Read the model definition and answer for the solid it produces. Units are mm, in the model's axes. A direction names the side the tool comes from. Round coordinates to 2 decimals unless told otherwise and drop trailing zeros. Order: outer loops, then holes, each group sorted by start corner. A loop starts at its lowest first (then second) coordinate and runs counter-clockwise, first axis right, second up. Notation, with made-up numbers: M 66.5,-13 L 86.5,-13 A9 ccw 86.5,0 Z; hole C 23,24.5 d7. An arc over 180 degrees is marked long. Use one line per item in the form item = value. Start each with the question number.
from build123d import *

# Parameters (mm, degrees)
CHANFRO1_SIZE = 0.5
FILETE1_R     = 3


with BuildPart() as part:
    # Esboço1 → Revolução1 (revolve)
    with BuildSketch(Plane(origin=(0, 0, 0), x_dir=(0, 0, -1), z_dir=(1, 0, 0))):
        Polygon((23.5, 20), (20, 20), (9.495318128, -6), (14.495318128, -6), (25, 20), (29.5, 20), (29.5, 35), (21.5, 35), (21.5, 23), (23.5, 23), align=None)
    revolve(axis=Axis((0, 0, 0), (0, 1, 0)))

    # Chanfro1
    chanfro1_edges = [part.edges().sort_by_distance(p)[0] for p in [
        (0, 35, 29.5),
        (0, 20, 29.5),
    ]]
    chamfer(chanfro1_edges, length=CHANFRO1_SIZE)

    # Filete1
    filete1_edges = [part.edges().sort_by_distance(p)[0] for p in [
        (0, 20, 25),
    ]]
    fillet(filete1_edges, radius=FILETE1_R)


solid = part.part
Item 1: Section C-C (y = 13.5) is taken. Write down the section's boundary in (x, z).
Item 2: Given P1, Ø23.5, axis at x = 1.5, z = -2, coming from the -Y side; P2, Ø8, axis at y = 0.5, z = 15, coming from the -X side; P3, Ø12, axis at x = -14, z = -4.5, coming from the +Y side; P4, Ø5, axis at x = -16, z = -4, coming from the +Y side, each flat-ended and moving along its own axis, determine where each tip first touches the part or whether it passes through.
Item 3: For a pull along Z with two mould halves and no side action, classify faces 3 (the flat face through (-13, 20, -24)), 4 (the cylindrical face through (-21.317, 28.916, 2.799)), 5 (the cylindrical face through (-8.86, 27.6, -28.14)) as pulls with the +Z half, pulls with the -Z half, needs draft (parallel to the pull), parting line crosses it, or undercut.
Item 4: Section A-A (z = 0) is taken. Write down the section's boundary in (x, y), and give its area (3 significant figures).
Item 5: Find the intervals of material crossed by L1, parallel to Z at x = 0, y = 21; L2, parallel to X at y = 28.5, z = 0, in increasing order. Write a range as [from, to].
Item 6: Section B-B (x = 0) is taken. Write down the section's boundary in (y, z), and give its area (3 significant figures).
Item 7: A tool of negligible diameter and unlimited length cuts with its end or side. For faces 1 (the cylindrical face through (-7.1, 21.5, -22.4)), 2 (the conical face through (-3.71, 1.04, -11.77)), from which of +Z, -Z, +X, -X, +Y, -Y can it reach the whole face along a straight path? Write none if from no direction.
Item 8: Section D-D (y = 4) is taken. Write down the section's boundary in (x, z).
The answers:
q1.outline = C 0,0 d44.75; hole C 0,0 d34.75
q2.P1 = -6
q2.P2 = -13.73
q2.P3 = 20
q2.P4 = 17.51
q3.face_3 = needs draft
q3.face_4 = undercut
q3.face_5 = parting line crosses it
q4.outline = M -29.5,20.5 L -29,20 L -27.02,20 A3 cw -24.24,18.12 L -14.5,-6 L -9.5,-6 L -20,20 L -23.5,20 L -23.5,23 L -21.5,23 L -21.5,35 L -29,35 L -29.5,34.5 Z; M 9.5,-6 L 14.5,-6 L 24.24,18.12 A3 cw 27.02,20 L 29,20 L 29.5,20.5 L 29.5,34.5 L 29,35 L 21.5,35 L 21.5,23 L 23.5,23 L 23.5,20 L 20,20 Z
q4.area = 489 mm²
q5.L1 = [-29.5, -23.5], [23.5, 29.5]
q5.L2 = [-29.5, -21.5], [21.5, 29.5]
q6.outline = M -6,-14.5 L 18.12,-24.24 A3 cw 20,-27.02 L 20,-29 L 20.5,-29.5 L 34.5,-29.5 L 35,-29 L 35,-21.5 L 23,-21.5 L 23,-23.5 L 20,-23.5 L 20,-20 L -6,-9.5 Z; M -6,9.5 L 20,20 L 20,23.5 L 23,23.5 L 23,21.5 L 35,21.5 L 35,29 L 34.5,29.5 L 20.5,29.5 L 20,29 L 20,27.02 A3 cw 18.12,24.24 L -6,14.5 Z
q6.area = 489 mm²
q7.face_1 = none
q7.face_2 = +Y
q8.outline = C 0,0 d37.07; hole C 0,0 d27.07
